Build history of the part. All positions in model axes, mm. A direction names the side the tool comes from. Give positions to 0.01 mm unless a question says otherwise; leave off trailing zeros. Order: outer loops, then holes, each group sorted by start corner. A loop starts at its lowest first (then second) coordinate and runs counter-clockwise, first axis right, second up. Notation, with made-up numbers: (-21.75, 48.25) -> (20.25, 48.25) arc R21 ccw to (20.25, 86.25) -> close; hole circle Ø6 at (33, -8). An arc over 180 degrees is marked (long way). Use a Markdown table: item, result. Add a question column.
```python
from build123d import *

# Parameters (mm, degrees)
F2_R     = 7.9375
F1_R     = 19.05
F4_R     = 4.2545
F5_DEPTH = 22.225
F6_DEPTH = 28.575
F7_R     = 15.870198
F8_DEPTH = 28.575


with BuildPart() as f3:
    # F2 (on Top) → F3 section 0
    with BuildSketch(Plane.XY):
        Circle(F2_R)
    # F1 (on offset) → F3 section 1
    with BuildSketch(Plane.XY.offset(22.225)):
        Circle(F1_R)
    loft()

    # F4 (on offset) → F5 (cut)
    with BuildSketch(Plane.XY.offset(22.225)):
        Circle(F4_R)
    extrude(amount=-F5_DEPTH, mode=Mode.SUBTRACT)

    # F1 (on offset) → F6 (join)
    with BuildSketch(Plane.XY.offset(22.225)):
        Circle(F1_R)
    extrude(amount=F6_DEPTH)

    # F7 (on face) → F8 (cut)
    with BuildSketch(Plane.XY.offset(50.8)):
        Circle(F7_R)
    extrude(amount=-F8_DEPTH, mode=Mode.SUBTRACT)


solid = f3.part
```
(1) Pin check, flat tips, straight feed: pin 1 Ø2 at (x, z) = (11.5, 42.5) entering from +Y; pin 2 Ø5 at (x, z) = (4, 31) entering from +Y; pin 3 Ø10 at (x, y) = (0, 0) entering from +Z (3 decimals). Stop position of each tip, or through.
(2) Mould opens along Y. For faces 1 (the face through (-8.81, -6.76, 6.33)), 2 (the face through (-4, 16, 50.8)), 3 (the face through (-15.855, 0.698, 36.713)) say: released by +Y, released by -Y, zero draft, split by the parting line, or undercut.
(3) Tool access for faces 4 (the face through (3.3, -3.3, 22.225)), 5 (the face through (-15.12, -11.59, 36.31)): list every direction of +Z, -Z, +X, -X, +Y, -Y with a clear straight run to the whole face (end or side of a thin tool).
(4) Band-saw the part on B-B on z = 9. Give the cut face in (x, y) (1 decimal).
(5) Wall check: probe 1 along Y at (x, z) = (0, 41.25); probe 2 along Y at (x, z) = (14, 29.5); probe 3 along Z at (x, y) = (5, -3) (3 decimals). Give the ranges that are in metal, low to high.
Response:
| question | item | result |
|---|---|---|
| 1 | pin 1 | stops at y = 15.9 |
| 1 | pin 2 | stops at y = 18.99 |
| 1 | pin 3 | stops at z = 22.225 |
| 2 | face 1 | split by the parting line |
| 2 | face 2 | zero draft |
| 2 | face 3 | undercut |
| 3 | face 4 | +Z |
| 3 | face 5 | +Z, -Z |
| 4 | outline | circle Ø24.9 at (0, 0); hole circle Ø8.5 at (0, 0) |
| 5 | probe 1 | y = -19.05 to -15.87, 15.87 to 19.05 |
| 5 | probe 2 | y = -12.92 to -7.47, 7.47 to 12.92 |
| 5 | probe 3 | z = 0 to 22.225 |
